```python
from build123d import *

# Parameters (mm, degrees)
F0_R     = 0.625
F1_DEPTH = 1.5


with BuildPart() as f1:
    # F0 (on Top) → F1 (new body)
    with BuildSketch(Plane.XY):
        with BuildLine():
            Line((-3.175, 0), (0, 0))
            Line((0, 0), (0, -1.5))
            Line((0, -1.5), (7, -1.5))
            Line((7, -1.5), (7, 0))
            Line((7, 0), (8.5, 0))
            Line((8.5, 0), (10.520726, 3.5))
            ThreePointArc((10.520726, 3.5), (12.350853, 5.330127), (14.850853, 6))
            Line((14.850853, 6), (15.25, 6))
            ThreePointArc((15.25, 6), (16.133883, 6.366117), (16.5, 7.25))
            Line((16.5, 7.25), (16.5, 8.75))
            ThreePointArc((16.5, 8.75), (16.133883, 9.633883), (15.25, 10))
            Line((15.25, 10), (10.562387, 10))
            ThreePointArc((10.562387, 10), (8.852286, 9.698463), (7.348449, 8.830222))
            Line((7.348449, 8.830222), (-3.175, 0))
        make_face()
        with Locations((14.5, 8)):
            Circle(F0_R, mode=Mode.SUBTRACT)
    extrude(amount=F1_DEPTH)


solid = f1.part
```
Could you check a few things on this model? Use its own coordinates, in mm. A direction names the side the tool comes from. Round coordinates to 2 decimals unless told otherwise and drop trailing zeros. Loops run counter-clockwise (first coordinate to the right, second up) from the corner with the lowest first, then second, coordinate; pieces in that order, holes last. Notation, with made-up numbers: (-17.75, 69) - (-9.75, 69) arc R21 ccw to (-9.75, 78) - close; hole circle Ø4 at (63, -12). An arc over 180 degrees is marked (long way). Answer as CSV lines item,"result".
1. On a 3-axis mill with a long thin cutter (end or side, diameter ignored), from which of +Z, -Z, +X, -X, +Y, -Y can I reach the whole of each face in a straight line? I mean faces 1 (the face through (8, 0, 1)), 2 (the face through (-2, 0, 1)), 3 (the face through (13, 10, 1)). Say none if no direction works.
Filled in:
face 1,"+Z, -Z, +X, -Y"
face 2,"+Z, -Z, -X, -Y"
face 3,"+Z, -Z, +X, -X, +Y"
2. I want a section at B-B on y = 8. List the corners of the cut face in (x, z) for me (3 decimals).
Filled in:
outline,"(6.359, 0) - (13.875, 0) - (13.875, 1.5) - (6.359, 1.5) - close; (15.125, 0) - (16.5, 0) - (16.5, 1.5) - (15.125, 1.5) - close"
3. We'd pull the mould along Y, two halves only. Please class faces 4 (the face through (8.88, 9.71, 0.74)), 5 (the face through (0, -1, 1)), 6 (the face through (14.836, 8.527, 0.74)): +Y half, -Y half, draft (parallel to the pull), parting line (faces both ways), or undercut.
Filled in:
face 4,"+Y half"
face 5,"draft"
face 6,"undercut"
4. I want a section at A-A on z = 0.85. List the corners of the cut face in (x, y) for me (3 decimals), then the cut area to 3 significant figures.
Filled in:
outline,"(-3.175, 0) - (0, 0) - (0, -1.5) - (7, -1.5) - (7, 0) - (8.5, 0) - (10.521, 3.5) arc R5 cw to (14.851, 6) - (15.25, 6) arc R1.25 ccw to (16.5, 7.25) - (16.5, 8.75) arc R1.25 ccw to (15.25, 10) - (10.562, 10) arc R5 ccw to (7.348, 8.83) - close; hole circle Ø1.25 at (14.5, 8)"
area,"109 mm^2"
5. I want a section at D-D on x = 0.5. List the corners of the cut face in (y, z) for me, then the cut area to 3 significant figures.
Filled in:
outline,"(-1.5, 0) - (3.08, 0) - (3.08, 1.5) - (-1.5, 1.5) - close"
area,"6.88 mm^2"
6. For pin 1 Ø0.8 at (x, y) = (14.5, 8) entering from -Z; pin 2 Ø0.8 at (y, z) = (-0.5, 0.5) entering from +X, each with a flat end and sliding along its axis, tell me the tip position at first contact or that it passes through.
Filled in:
pin 1,"passes through"
pin 2,"stops at x = 7"
7. Please list where these lines run through material, in increasing order: line 1 along Y through (x, z) = (14.5, 1.1) (3 decimals); line 2 along X through (y, z) = (4, 1.2); line 3 along X through (y, z) = (7.75, 0.65). Write a range as [from, to].
Filled in:
line 1,"y = [5.988, 7.375], [8.625, 10]"
line 2,"x = [1.59, 10.85]"
line 3,"x = [6.06, 13.93], [15.07, 16.5]"
8. I want a section at C-C on x = 14.5. List the corners of the cut face in (y, z) for me (3 decimals).
Filled in:
outline,"(5.988, 0) - (7.375, 0) - (7.375, 1.5) - (5.988, 1.5) - close; (8.625, 0) - (10, 0) - (10, 1.5) - (8.625, 1.5) - close"
